from build123d import *

# Parameters (mm, degrees)
SKETCH1_W               = 15.875
SKETCH1_H               = 15.875
BOSS_EXTRUDE1_DEPTH     = 53.975
CUT_EXTRUDE1_DEPTH      = 57.818308284
CUT_EXTRUDE1_DEPTH_BACK = 57.818308284
F_12_24_TAPPED_HOLE1_D  = 4.4958


with BuildPart() as part:
    # Sketch1 → Boss-Extrude1 (new, symmetric)
    with BuildSketch(Plane.XY):
        Rectangle(SKETCH1_W, SKETCH1_H)
    extrude(amount=BOSS_EXTRUDE1_DEPTH, both=True)

    # Sketch2 → Cut-Extrude1 (cut, two sides: drawn at the far end of the back side and taken through both)
    with BuildSketch(Plane(origin=(0, 7.9375, 0), x_dir=(1, 0, 0), z_dir=(0, 1, 0)).offset(-CUT_EXTRUDE1_DEPTH_BACK)):
        Polygon((71.794217754, 150.202262663), (7.9375, 14.2875), (5.699938661, 9.525), (7.9375, 4.7625), (71.794217754, -131.152262663), (372.130716448, -131.152262663), (372.130716448, 150.202262663), align=None)
    extrude(amount=CUT_EXTRUDE1_DEPTH + CUT_EXTRUDE1_DEPTH_BACK, mode=Mode.SUBTRACT)

    # #12-24 Tapped Hole1 (through all)
    with Locations(Plane(origin=(7.9375, 0, 0), x_dir=(0, 0, -1), z_dir=(1, 0, 0))):
        with Locations((38.1, 0), (-19.05, 0)):
            Hole(F_12_24_TAPPED_HOLE1_D / 2)


solid = part.part
Here's how the part is built. I have some questions about the finished solid (model axes, mm). A direction names the side the tool comes from. Round coordinates to 2 decimals unless told otherwise and drop trailing zeros. Loops run counter-clockwise (first coordinate to the right, second up) from the corner with the lowest first, then second, coordinate; pieces in that order, holes last.
1. If we section it at C-C on x = -2.25: Count the separate pieces of the cut face and the enclosed holes in it, plus the area to 3 significant figures.
Answer list:
separate pieces: 1
enclosed holes: 2
area: 1,680 mm2
2. If I drill on line 1 along Y through (x, z) = (-0.25, 19.05); line 2 along Z through (x, y) = (-3.5, 0.5) (3 decimals); line 3 along Z through (x, y) = (-1, 1.75) (3 decimals), over which ranges is the centre line in solid material (lowest first)?
Answer list:
line 1: y = -7.94 to -2.25, 2.25 to 7.94
line 2: z = -53.975 to -40.292, -35.908 to 16.858, 21.242 to 53.975
line 3: z = -53.975 to -39.511, -36.689 to 17.639, 20.461 to 53.975
3. We'd pull the mould along Y, two halves only. Please class faces 1 (the face through (-7.938, 0, 1)), 2 (the face through (-0.111, 0.675, 21.194)), 3 (the face through (0, 7.938, 1)): +Y half, -Y half, draft (parallel to the pull), parting line (faces both ways), or undercut.
Answer list:
face 1: draft
face 2: undercut
face 3: +Y half
4. If we section it at A-A on y = 0: Write out the boundary of the cut face in (x, z) (1 decimal), plus the area to 3 significant figures.
Answer list:
outline: (-7.9, -54) - (7.9, -54) - (7.9, -40.3) - (-7.9, -40.3) - close; (-7.9, -35.9) - (7.9, -35.9) - (7.9, -14.3) - (5.7, -9.5) - (7.9, -4.8) - (7.9, 16.8) - (-7.9, 16.8) - close; (-7.9, 21.3) - (7.9, 21.3) - (7.9, 54) - (-7.9, 54) - close
area: 1,560 mm2
5. If we section it at D-D on z = -7.5: Write out the boundary of the cut face in (x, y).
Answer list:
outline: (-7.94, -7.94) - (6.65, -7.94) - (6.65, 7.94) - (-7.94, 7.94) - close
6. If we section it at B-B on z = 19.05: Write out the boundary of the cut face in (x, y).
Answer list:
outline: (-7.94, -7.94) - (7.94, -7.94) - (7.94, -2.25) - (-7.94, -2.25) - close; (-7.94, 2.25) - (7.94, 2.25) - (7.94, 7.94) - (-7.94, 7.94) - close
7. Which directions (+Z, -Z, +X, -X, +Y, -Y) give clear straight access to the entire face, cutting with the end or side of a thin tool? Please do faces 4 (the face through (6.834, -0.111, -11.94)), 5 (the face through (7.938, 0, -34)).
Answer list:
face 4: +X, +Y, -Y
face 5: +Z, -Z, +X, +Y, -Y
